Input: part model. Units: mm. Frame: model coordinates. Face numbers are marked on the shaded views. A direction names the side the tool comes from. Give positions to 0.01 mm unless a question says otherwise; leave off trailing zeros. Loops run counter-clockwise (first coordinate to the right, second up) from the corner with the lowest first, then second, coordinate; pieces in that order, holes last.
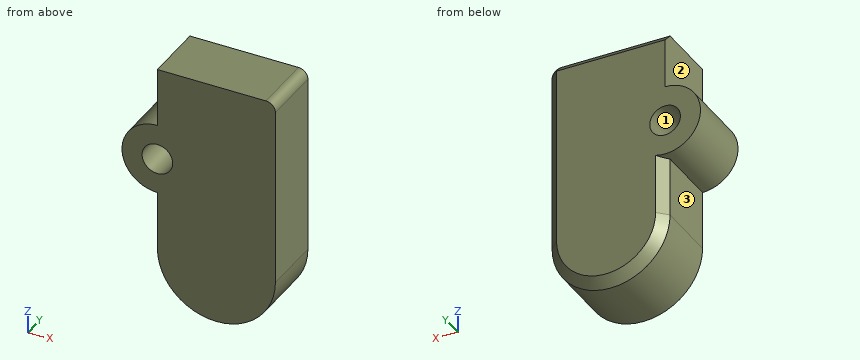
Autodesk Inventor part; units mm, degrees
ref_plane "YZ Plane" through (0, 0, 0) normal (1, 0, 0) x (0, 1, 0)
ref_plane "XZ Plane" through (0, 0, 0) normal (0, 1, 0) x (-1, 0, 0)
ref_plane "XY Plane" through (0, 0, 0) normal (0, 0, 1) x (1, 0, 0)
sketch "Sketch1" plane through (0, 0, 0) normal (0, 1, 0) x (-1, 0, 0)
  line L0 (-12.5, -20) -> (12.5, -20)
  line L1 (12.5, -20) -> (12.5, 20)
  line L2 (12.5, 20) -> (-12.5, 20)
  line L3 (-12.5, 20) -> (-12.5, -20)
  line L4 (-12.5, -20) -> (12.5, 20) construction
  line L5 (12.5, -20) -> (-12.5, 20) construction
  circle A0 centre (0, -20) radius 12.5
  circle A1 centre (12.5, 0) radius 7.5
  point P0 (0, 0)
  point P1 (12.5, -7.5)
  point P2 (12.5, 7.5)
  dimension "d0" = 25
  dimension "d1" = 40
  dimension "d2" = 15
extrude "Extrusion1" add sketch "Sketch1" along normal blind 15
fillet "Fillet1" radius 2 1 edges at (12.5, 7.5, 20)
chamfer "Chamfer1" distance 2 angle 45 5 edges at (-1, 15, 20) (11.9142, 15, 19.4142) (12.5, 15, -1) (0, 15, -32.5) (-12.5, 15, -13.75)
sketch "Sketch2" plane through (0, 15, 0) normal (0, 1, 0) x (1, 0, 0)
  arc A0 (-10.5, 7.2284) -> (-12.5, -7.5) centre (-12.5, 0) ccw
  point P0 (0, 0)
hole "Hole1" at (-12.5, 15, 0) direction (0, -1, 0) diameter 6.5 end through all
equation "\"d3\" = d2"
properties part number "SampleComplexPart"
(1) Cut plane C-C (z = 12.5). Return the cut outline in (x, y).
Values follow:
outline: (-12.5, 0) - (12.5, 0) - (12.5, 13) - (10.5, 15) - (-12.5, 15) - close
(2) Ray query, probe 1 along X at (y, z) = (10, 0); probe 2 along X at (y, z) = (8, 14.5); probe 3 along Z at (x, y) = (0, 4). Return the intervals inside material, ascending.
Values follow:
probe 1: x = -20 to -15.75, -9.25 to 12.5
probe 2: x = -12.5 to 12.5
probe 3: z = -32.5 to 20
(3) Pin query (flat end, axial travel): pin 1 Ø4 at (y, z) = (7, -21) entering from -X; pin 2 Ø2 at (x, y) = (-2.5, 11) entering from -Z; pin 3 Ø4 at (x, z) = (-12.5, 0) entering from +Y. Return the tip coordinate at first contact, or that it passes through.
Values follow:
pin 1: stops at x = -12.5
pin 2: stops at z = -32.41
pin 3: passes through
(4) Reachability of the marked faces 1, 2 and 3 from +Z, -Z, +X, -X, +Y, -Y: full face, straight path, thin tool, end or side. Return the list, or none.
Values follow:
face 1: +Y, -Y
face 2: +Z, -X, +Y, -Y
face 3: -Z, -X, +Y, -Y
(5) Cut plane A-A (z = 0). Return the cut outline in (x, y), and give its area (3 significant figures).
Values follow:
outline: (-20, 0) - (-15.75, 0) - (-15.75, 15) - (-20, 15) - close; (-9.25, 0) - (12.5, 0) - (12.5, 13) - (10.5, 15) - (-9.25, 15) - close
area: 388 mm2
(6) Cut plane D-D (z = 5.5). Return the cut outline in (x, y).
Values follow:
outline: (-17.6, 0) - (12.5, 0) - (12.5, 13) - (10.5, 15) - (-17.6, 15) - close
(7) Cut plane B-B (y = 5.25). Return the cut outline in (x, z).
Values follow:
outline: (-12.5, -20) arc R12.5 ccw to (12.5, -20) - (12.5, 18) arc R2 ccw to (10.5, 20) - (-12.5, 20) - (-12.5, 7.5) arc R7.5 ccw to (-12.5, -7.5) - close; hole circle Ø6.5 at (-12.5, 0)
